The model under review builds one solid part; all positions refer to its coordinate system, in mm. A direction names the side the tool comes from. Round coordinates to 2 decimals unless told otherwise and drop trailing zeros. Order: outer loops, then holes, each group sorted by start corner. A loop starts at its lowest first (then second) coordinate and runs counter-clockwise, first axis right, second up. Notation, with made-up numbers: (-18.5, 35) - (1.5, 35) arc R23 ccw to (1.5, 49) - close; hole circle Ø2 at (-17.75, 28.25). An arc over 180 degrees is marked (long way). One line per question, with ' | ' between items. Start each with the question number.
Item 1: Add section B-B on z = -29.4. State how many separate pieces and enclosed holes the cut face has, and give its area (3 significant figures).
Item 2: Draft analysis for pull direction Z (two halves, no side actions). For faces 4 (the face through (176.5, 18, -6.7)), 5 (the face through (304.9, 0.6, -20.4)), 6 (the face through (95, 4, -1.2)), 7 (the face through (95, 4, -20.4)), state which applies: +Z half, -Z half, draft (parallel to the pull), parting line (faces both ways), or undercut.
Item 3: For L1, parallel to X at y = 16, z = -21.5; L2, parallel to X at y = 15, z = -49.5; L3, parallel to X at y = 4.75, z = -27, list the stretches that pass through material, from the lowest coordinate up. Write a range as [from, to].
Item 4: Insertion check: pin 1 Ø21 at (x, z) = (37, -68.5) entering from +Y; pin 2 Ø5 at (x, y) = (65.5, 2.5) entering from -Z; pin 3 Ø1.3 at (y, z) = (6, -77.5) entering from +X. Each pin has a flat end and moves straight along its axis. Give the tip position at first contact, or say it passes through.
Item 5: Tool access review of faces 1 (the face through (20.402, 3.971, -29.598)), 2 (the face through (63.934, 2.566, -77.432)), 3 (the face through (43.153, 4.437, -63.386)): name each direction out of +Z, -Z, +X, -X, +Y, -Y from which nothing blocks a thin tool from reaching the whole face with its end or side.
Item 6: Add section A-A on y = 15. State the section outline as (x, z) points, and give its area (3 significant figures).
Autodesk Inventor part; units mm, degrees
ref_plane "YZ Plane" through (0, 0, 0) normal (1, 0, 0) x (0, 1, 0)
ref_plane "XZ Plane" through (0, 0, 0) normal (0, 1, 0) x (-1, 0, 0)
ref_plane "XY Plane" through (0, 0, 0) normal (0, 0, 1) x (1, 0, 0)
sketch "Esboço1" plane through (0, 0, 0) normal (0, 1, 0) x (-1, 0, 0)
  arc A0 (-292.0445, -21.6) -> (-182.0445, -21.6) centre (-237.0445, -21.6) ccw
  line L0 (-292.0445, -21.6) -> (-237.0445, -21.6) construction
  line L1 (-182.0445, -21.6) -> (-237.0445, -21.6) construction
  arc A1 (-161.6445, -1.2) -> (-182.0445, -21.6) centre (-161.6445, -21.6) ccw
  line L2 (-182.0445, -21.6) -> (-161.6445, -21.6) construction
  line L3 (-161.6445, -1.2) -> (-161.6445, -21.6) construction
  arc A2 (-29.4, -57.6) -> (-29.4, -1.2) centre (-29.4, -29.4) ccw
  line L4 (-29.4, -1.2) -> (-29.4, -29.4) construction
  line L5 (-29.4, -57.6) -> (-29.4, -29.4) construction
  arc A3 (-29.4, -57.6) -> (-48.64, -76.8399) centre (-29.4, -76.8399) ccw
  line L6 (-29.4, -57.6) -> (-29.4, -76.8399) construction
  line L7 (-48.64, -76.8399) -> (-29.4, -76.8399) construction
  line L8 (-29.4, -1.2) -> (-161.6445, -1.2)
  arc A4 (-310.0445, -21.6) -> (-164.0445, -21.6) centre (-237.0445, -21.6) ccw
  arc A5 (-161.6445, -19.2) -> (-164.0445, -21.6) centre (-161.6445, -21.6) ccw
  line L9 (-161.6445, -19.2) -> (-29.4, -19.2)
  arc A6 (-29.4, -39.6) -> (-29.4, -19.2) centre (-29.4, -29.4) ccw
  arc A7 (-29.4, -39.6) -> (-66.64, -76.8399) centre (-29.4, -76.8399) ccw
  line L10 (-48.64, -76.8399) -> (-66.64, -76.8399)
  line L11 (-292.0445, -21.6) -> (-310.0445, -21.6)
  arc A8 (-311.2348, -20.4) -> (-162.8445, -21.6) centre (-237.0445, -21.6) ccw
  line L12 (-311.2348, -20.4) -> (-290.8311, -20.4)
  arc A9 (-290.8311, -20.4) -> (-183.2445, -21.6) centre (-237.0445, -21.6) ccw
  arc A10 (-161.6445, 0) -> (-183.2445, -21.6) centre (-161.6445, -21.6) ccw
  line L13 (-161.6445, 0) -> (-29.4, 0)
  arc A11 (-29.4, -58.8) -> (-29.4, 0) centre (-29.4, -29.4) ccw
  arc A12 (-29.4, -58.8) -> (-47.4, -78.0399) centre (-29.4, -76.8399) ccw
  line L14 (-47.4, -78.0399) -> (-67.8212, -78.0399)
  arc A13 (-29.4, -38.4) -> (-67.8212, -78.0399) centre (-29.4, -76.8399) ccw
  arc A14 (-29.4, -38.4) -> (-29.4, -20.4) centre (-29.4, -29.4) ccw
  line L15 (-29.4, -20.4) -> (-161.6445, -20.4)
  arc A15 (-161.6445, -20.4) -> (-162.8445, -21.6) centre (-161.6445, -21.6) ccw
  line L16 (-66.64, -76.8399) -> (-66.64, -78.0399)
  line L17 (-48.64, -78.0399) -> (-48.64, -76.8399)
  line L18 (-310.0445, -21.6) -> (-310.0445, -20.4)
  line L19 (-292.0445, -21.6) -> (-292.0445, -20.4)
  line L20 (-164.0445, -21.6) -> (-162.8445, -21.6)
  line L21 (-182.0445, -21.6) -> (-183.2445, -21.6)
  line L22 (-161.6445, -1.2) -> (-161.6445, 0)
  line L23 (-161.6445, -20.4) -> (-161.6445, -19.2)
  line L24 (-29.4, -38.4) -> (-29.4, -39.6)
  line L25 (-29.4, -57.6) -> (-29.4, -58.8)
  line L26 (-29.4, -1.2) -> (-29.4, 0)
  point P0 (0, 0)
  point P1 (-163.4445, -21.6)
  point P2 (-95.5222, 0)
  point P3 (0, -29.4)
  point P4 (-95.5222, -20.4)
  point P5 (-301.0329, -20.4)
  point P6 (-161.6445, -0.6)
  point P7 (-182.6445, -21.6)
  point P8 (-161.6445, -19.8)
  point P9 (-183.2445, -21.6)
  point P10 (-182.0445, -21.6)
  point P11 (-161.6445, 0)
  point P12 (-161.6445, -1.2)
  point P13 (-164.0445, -21.6)
  point P14 (-162.8445, -21.6)
  point P15 (-29.4, -39)
  point P16 (-29.4, -58.2)
  point P17 (-29.4, -0.6)
  point P18 (-29.4, -58.8)
  point P19 (-29.4, -57.6)
  point P20 (-29.4, -1.2)
  point P21 (-29.4, 0)
  dimension "d22" = 180
  dimension "d23" = 110
  dimension "d24" = 90
  dimension "d25" = 180
  dimension "d26" = 90
  dimension "d27" = 18
  dimension "d28" = 18
  dimension "d29" = 18
  dimension "d30" = 20.4
  dimension "d31" = 1.2
  dimension "d32" = 18
  dimension "d33" = 132.2445
extrude "Extrusão1" add sketch "Esboço1" against normal blind 1.2
extrude "Extrusão2" add sketch "Esboço1" along normal blind 9 contours L19 L12 A9 L21 A0 | L22 L13 L26 L8 | A5 L23 A15 L20 | L9 A6 L24 A14 L15 L23 | L25 A12 L14 L17 A3 | A7 L16 L14 A13 L24
extrude "Extrusão3" add sketch "Esboço1" along normal blind 18 contours L21 A10 L22 A1 | A4 L20 A8 L12 L18 | L26 A11 L25 A2
fillet "Arredondamento2" radius 9 7 edges at (19.2, 0, -29.4) (55.7326, 0, -50.5073) (66.64, 0, -77.4399) (163.3415, 0, -19.9029) (237.0445, 0, -94.6) (310.0445, 0, -21) (95.5222, 0, -19.2)
equation "\"d27\" = Diâmetro_esfera"
equation "\"d28\" = Diâmetro_esfera"
equation "\"d29\" = Diâmetro_esfera"
equation "\"Diâmetro_esfera\" = 18"
equation "\"Filamento\" = 0.4"
equation "\"Margem\" = 3 * Filamento"
equation "\"Parafuso\" = 3"
properties part number "Agrupar bolinhas novamente" material "Plástico PET"
Determined:
1) separate pieces: 3 | enclosed holes: 0 | area: 224 mm2
2) face 4: draft | face 5: +Z half | face 6: undercut | face 7: undercut
3) L1: [1.08, 2.33], [182.04, 183.24], [310.04, 311.24] | L2: [7.94, 9.62], [168.29, 169.59], [304.5, 305.8] | L3: [0.1, 1.3], [18.39, 20.73], [163.04, 165.31], [182.31, 183.52], [290.57, 291.78], [308.78, 311.05]
4) pin 1: y = 9 | pin 2: z = -78.04 | pin 3: x = 286.57
5) face 1: +Y, -Y | face 2: -Z, +Y | face 3: +Y
6) outline: (29.4, -58.8) - (29.4, -57.6) arc R28.2 cw to (29.4, -1.2) - (29.4, 0) arc R29.4 ccw to start; (161.64, -1.2) arc R20.4 cw to (182.04, -21.6) - (183.24, -21.6) arc R21.6 ccw to (161.64, 0) - close; (162.84, -21.6) arc R74.2 ccw (long way) to (311.23, -20.4) - (310.04, -20.4) - (310.04, -21.6) arc R73 cw to (164.04, -21.6) - close | area: 427 mm2
